Here's how the part is built. I have some questions about the finished solid (model axes, mm). Face numbers are marked on the shaded views. A direction names the side the tool comes from. Coordinates: 2 decimals unless noted, no trailing zeros. Order: outer loops, then holes, each group sorted by start corner. A loop starts at its lowest first (then second) coordinate and runs counter-clockwise, first axis right, second up. Notation, with made-up numbers: (78.25, 76.25) - (119.25, 76.25) arc R29 cw to (119.25, 98.25) - close; hole circle Ø3 at (53.5, -4). An arc over 180 degrees is marked (long way). Use CSV: the item, a comma, the result in double quotes. Start each with the question number.
Autodesk Fusion 360 part; units mm, degrees
sketch "Sketch1" plane through (0, 0, 0) normal (1, 0, 0) x (0, 1, 0)
  line L0 (0, 0) -> (0, 45)
  line L1 (0, 0) -> (0, -45)
  line L2 (0, 45) -> (37.5, 45)
  line L3 (0, 45) -> (-37.5, 45)
  line L4 (0, -45) -> (37.5, -45)
  line L5 (0, -45) -> (-37.5, -45)
  arc A0 (-37.5, 45) -> (-37.5, -45) centre (79.119, 0) ccw
  arc A1 (37.5, -45) -> (37.5, 45) centre (-79.119, 0) ccw
  dimension "d1" = 37.5
  dimension "d2" = 37.5
  dimension "d3" = 37.5
  dimension "d4" = 37.5
  dimension "d5" = 125
  dimension "d6" = 125
extrude "Extrude1" add sketch "Sketch1" along normal blind 100
extrude "Extrude2" add 1 faces at (100, -14.2806, -15.2642) along direction (1, 0, 0) blind 35 draft -15
sketch "Sketch2" plane through (135, 0, 0) normal (1, 0, 0) x (0, 1, 0)
  line L0 (-30.8786, -35.6218) -> (30.8786, -35.6218)
  arc A0 (30.8786, -35.6218) -> (30.8786, 35.6218) centre (-79.119, 0) ccw
  line L1 (30.8786, 35.6218) -> (-30.8786, 35.6218)
  arc A1 (-30.8786, 35.6218) -> (-30.8786, -35.6218) centre (79.119, 0) ccw
  circle A2 centre (0, 0) radius 34.5
  dimension "d11" = 69
extrude "Extrude3" add sketch "Sketch2" along normal blind 10 contours A2
sketch "Sketch3" plane through (145, 0, 0) normal (1, 0, 0) x (0, 1, 0)
  circle A0 centre (0, 0) radius 34.5
  circle A1 centre (0, 0) radius 31
  dimension "d14" = 62
extrude "Extrude4" add sketch "Sketch3" along normal blind 30 contours A1
sketch "Sketch4" plane through (175, 0, 0) normal (1, 0, 0) x (0, 1, 0)
  circle A0 centre (0, 0) radius 31
  line L0 (0, 0) -> (27, 0)
  circle A1 centre (27, 0) radius 2.5
  circle A2 centre (27, 0) radius 1.5
  dimension "d17" = 27
  dimension "d18" = 5
  dimension "d19" = -1
extrude "Extrude5" add sketch "Sketch4" along normal blind 1 contours A1
pattern_circular "C-Pattern1" count 12 over 360 about axis through (175, 0, 0) along (1, 0, 0) of "Extrude5"
sketch "Sketch5" plane through (175, 0, 0) normal (1, 0, 0) x (0, 1, 0)
  circle A0 centre (13.5, -23.3827) radius 2.5
  circle A1 centre (-13.5, -23.3827) radius 2.5
  circle A2 centre (-27, 0) radius 2.5
  circle A3 centre (-13.5, 23.3827) radius 2.5
  circle A4 centre (13.5, 23.3827) radius 2.5
  circle A5 centre (27, 0) radius 2.5
  circle A6 centre (0, 0) radius 31
  circle A7 centre (23.3827, 13.5) radius 2.5
  circle A8 centre (0, 27) radius 2.5
  circle A9 centre (-23.3827, 13.5) radius 2.5
  circle A10 centre (-23.3827, -13.5) radius 2.5
  circle A11 centre (0, -27) radius 2.5
  circle A12 centre (23.3827, -13.5) radius 2.5
  line L0 (16, 0) -> (16, 17)
  line L1 (16, 0) -> (16, -17)
  line L2 (-16, 0) -> (-16, 17)
  line L3 (-16, 0) -> (-16, -17)
  arc A13 (-16, -17) -> (16, -17) centre (0, -1.9003) ccw
  arc A14 (16, 17) -> (-16, 17) centre (0, 1.9003) ccw
  dimension "d32" = 22
  dimension "d33" = 17
  dimension "d34" = 17
extrude "Extrude6" add sketch "Sketch5" along normal blind 100 contours L0 L1 L2 L3 A13 A14
sketch "Sketch6" plane through (275, 0, 0) normal (1, 0, 0) x (0, 1, 0)
  line L0 (16, -17) -> (16, 17)
  arc A0 (16, 17) -> (-16, 17) centre (0, 1.9003) ccw
  line L1 (-16, 17) -> (-16, -17)
  arc A1 (-16, -17) -> (16, -17) centre (0, -1.9003) ccw
  circle A2 centre (0, 0) radius 31
  dimension "d37" = 62
extrude "Extrude7" add sketch "Sketch6" along normal blind 10 contours L0 A0 L1 A1 | A2
sketch "Sketch7" plane through (285, 0, 0) normal (1, 0, 0) x (0, 1, 0)
  circle A0 centre (0, 0) radius 31
  circle A1 centre (0, 0) radius 30
  dimension "d40" = -1
extrude "Extrude8" add sketch "Sketch7" along normal blind 1
sketch "Sketch8" plane through (285, 0, 0) normal (1, 0, 0) x (0, 1, 0)
  circle A0 centre (0, 0) radius 30
  circle A1 centre (0, 0) radius 31
  dimension "d43" = 62
extrude "Extrude9" add sketch "Sketch8" along normal blind 10 contours A0
ref_plane "WorkPlane1" through (0, -37.5, 45) normal (0, -1, 0) x (1, 0, 0)
sketch "Sketch9" plane through (0, -37.5, 0) normal (0, -1, 0) x (-1, 0, 0)
  circle A0 centre (-50, 45) radius 42.5
  dimension "d46" = 85
extrude "Extrude10" add sketch "Sketch9" along normal mid plane 21
sketch "Sketch10" plane through (0, -27, 0) normal (0, 1, 0) x (-1, 0, 0)
  line L0 (-7.5, -45) -> (-92.5, -45)
  arc A0 (-92.5, -45) -> (-7.5, -45) centre (-50, -45) ccw
  line L1 (-50, -45) -> (-50, -75)
  line L2 (-70, -45) -> (-70, -77.2846)
  line L3 (-30, -45) -> (-30, -77.2846)
  arc A1 (-70, -77.2846) -> (-30, -77.2846) centre (-50, -54.924) ccw
  dimension "d49" = 30
  dimension "d50" = 20
  dimension "d51" = -20
  dimension "d52" = 30
extrude "Extrude11" add sketch "Sketch10" along normal blind 35 contours L0 L2 L3 A1
sketch "Sketch11" plane through (70, 0, 0) normal (1, 0, 0) x (0, 1, 0)
  line L0 (-27, -45) -> (-27, -77.2846)
  line L1 (-27, -77.2846) -> (8, -77.2846)
  line L2 (8, -77.2846) -> (8, -45)
  line L3 (8, -45) -> (-27, -45)
  line L4 (8, -45) -> (33, -45)
  line L5 (8, -45) -> (8, -87)
  arc A0 (8, -87) -> (33, -45) centre (-21.8393, -40.7981) ccw
  dimension "d55" = 25
  dimension "d56" = 42
  dimension "d57" = 55
extrude "Extrude12" add sketch "Sketch11" against normal blind 40 contours L2 L4 L5 A0
extrude "Extrude13" cut 1 faces at (33.5817, 8, -83.0165) along direction (0, 1, 0) blind 25
sketch "Sketch12" plane through (295, 0, 0) normal (1, 0, 0) x (0, 1, 0)
  circle A0 centre (0, 0) radius 30
  circle A1 centre (0, 0) radius 15
  dimension "d62" = 30
extrude "Extrude14" cut sketch "Sketch12" against normal blind 20 contours A1
sketch "Sketch13" plane through (0, -48, 0) normal (0, -1, 0) x (1, 0, 0)
  circle A0 centre (50, -45) radius 42.5
  circle A1 centre (50, -45) radius 15
  dimension "d65" = 30
extrude "Extrude15" cut sketch "Sketch13" against normal blind 20 contours A1
equation "d47 = ( 21 / 2 ) * 1 mm"
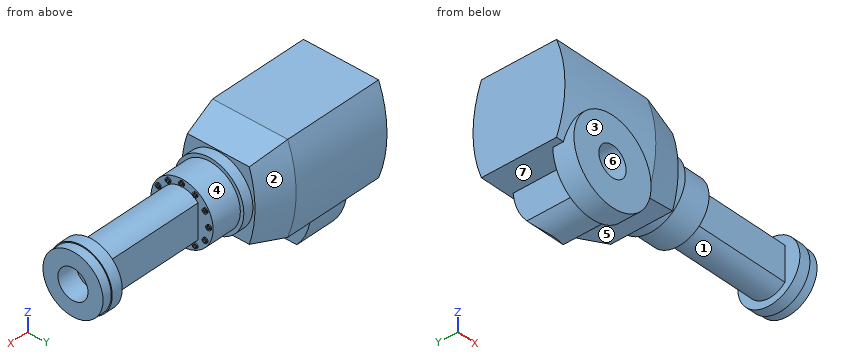
Item 1: Suppose I cut it at A-A on x = 96.5. Write out the boundary of the cut face in (y, z).
Item 2: For pin 1 Ø16 at (y, z) = (4, -58) entering from +X; pin 2 Ø12 at (x, y) = (131.5, 24.5) entering from +Z; pin 3 Ø1 at (x, z) = (90.5, 18) entering from -Y, each with a flat end and sliding along its axis, tell me the tip position at first contact or that it passes through.
Item 3: Please list where these lines run through material, in increasing order: line 1 along Y through (x, z) = (175.75, -13.5); line 2 along X through (y, z) = (-22, -53.5); line 3 along X through (y, z) = (8.5, -6.5). Write a range as from..to.
Item 4: For the marked faces 4, 5, 6 and 7, which set-ups out of +Z, -Z, +X, -X, +Y, -Y let a thin tool reach every point of the face, with its end or its side?
Item 5: We'd pull the mould along X, two halves only. Please class the marked faces 1, 2 and 3: released by +X, released by -X, zero draft, split by the parting line, or undercut.
Item 6: Suppose I cut it at B-B on x = 50. Write out the boundary of the cut face in (y, z), then the cut area to 3 significant figures.
Here are the results:
1,outline,"(-37.5, -45) - (37.5, -45) arc R125 ccw to (37.5, 45) - (-37.5, 45) arc R125 ccw to start"
2,pin 1,"x = 70"
2,pin 2,"z = 38.17"
2,pin 3,"y = -44.65"
3,line 1,"-25.88..-24.88, -21.88..-20.88, -16..16, 20.88..21.88, 24.88..25.88"
3,line 2,"30..70"
3,line 3,"0..275"
4,face 4,"+X"
4,face 5,"-Z, +X, +Y, -Y"
4,face 6,"-Y"
4,face 7,"-Z, +Y"
5,face 1,"undercut"
5,face 2,"released by +X"
5,face 3,"zero draft"
6,outline,"(-48, -87.5) - (-27, -87.5) - (-27, -84.92) - (10.99, -84.92) arc R55 ccw to (33, -45) - (37.5, -45) arc R125 ccw to (37.5, 45) - (-37.5, 45) arc R125 ccw to (-45.86, -2.5) - (-48, -2.5) - (-48, -30) - (-28, -30) - (-28, -60) - (-48, -60) - close"
6,area,"10,400 mm^2"
